The figure shows three views and two pictorial views of one solid part (mm, origin at its lowest corner). Answer the questions. A direction names the side the tool comes from. Round coordinates to 2 decimals unless told otherwise and drop trailing zeros. Write each loop counter-clockwise with the first axis right and the second up, starting at its lowest first coordinate (ties: lowest second). Pieces come first, ordered by that corner, then holes. Notation, with made-up numbers: M -18.5,24 L 27.5,24 A9 ccw 27.5,31 Z; hole C -9.5,42.5 d2. An arc over 180 degrees is marked long. One line per item, written item: value. Start each with the question number.
Q1. A tool of negligible diameter and unlimited length cuts with its end or side. For the marked faces 1 and 2, from which of +Z, -Z, +X, -X, +Y, -Y can it reach the whole face along a straight path? Write none if from no direction.
Q2. Consider probe 1 along Z at (x, y) = (7.25, 36.5) (1 decimal); probe 2 along Z at (x, y) = (6, 2) (1 decimal); probe 3 along Y at (x, z) = (1.75, 33) (1 decimal). Determine where each line is inside the solid, lowest interval first.
Q3. The mould has two halves that part along Y. Classify the marked faces 3, 4, 5 and 6: released by +Y, released by -Y, zero draft, split by the parting line, or undercut.
Q4. Given pin 1 Ø1.9 at (x, y) = (3.5, 1.5) entering from -Z (1 decimal); pin 2 Ø1.9 at (x, z) = (2.5, 48.5) entering from +Y (1 decimal); pin 3 Ø1.5 at (x, y) = (4.5, 25.5) entering from +Z, each flat-ended and moving along its own axis, determine where each tip first touches the part or whether it passes through.
Q5. Find section A-A (x = 4.25). Write down the section's boundary in (y, z), and give its area (3 significant figures).
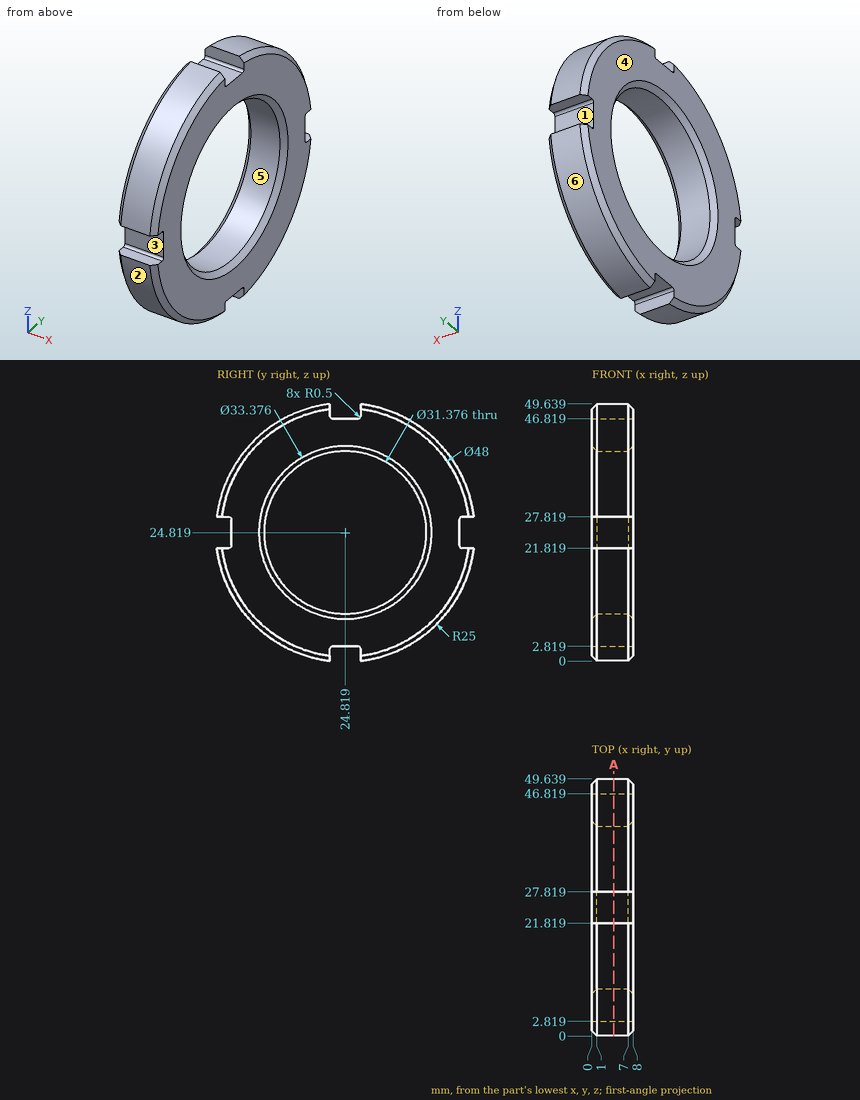
The answers:
1. face 1: +X, -X, +Y
1. face 2: -Z, +X, -X, -Y
2. probe 1: 3 to 14, 35.7 to 46.6
2. probe 2: 14.6 to 21.8, 27.8 to 35
2. probe 3: 1.2 to 11.4, 38.2 to 48.4
3. face 3: released by -Y
3. face 4: zero draft
3. face 5: undercut
3. face 6: released by +Y
4. pin 1: z = 13.7
4. pin 2: y = 35.2
4. pin 3: z = 46.82
5. outline: M 0,21.82 A25 ccw 21.82,0 L 21.82,2.32 A0.5 cw 22.32,2.82 L 27.32,2.82 A0.5 cw 27.82,2.32 L 27.82,0 A25 ccw 49.64,21.82 L 47.32,21.82 A0.5 cw 46.82,22.32 L 46.82,27.32 A0.5 cw 47.32,27.82 L 49.64,27.82 A25 ccw 27.82,49.64 L 27.82,47.32 A0.5 cw 27.32,46.82 L 22.32,46.82 A0.5 cw 21.82,47.32 L 21.82,49.64 A25 ccw 0,27.82 L 2.32,27.82 A0.5 cw 2.82,27.32 L 2.82,22.32 A0.5 cw 2.32,21.82 Z; hole C 24.82,24.82 d31.38
5. area: 1,120 mm2
